```python
from build123d import *

# Parameters (mm, degrees)
SKETCH1_R           = 4.625
SKETCH1_R_2         = 1.625
BOSS_EXTRUDE1_DEPTH = 10
SKETCH1_3_R         = 19.75
SKETCH1_3_R_2       = 18.75
SKETCH1_3_R_3       = 17.65
SKETCH1_3_R_4       = 4.625
SKETCH1_3_R_5       = 15.65
SKETCH1_3_R_6       = 1.625
BOSS_EXTRUDE2_DEPTH = 5
SKETCH1_4_R         = 19.75
SKETCH1_4_R_2       = 18.75
SKETCH1_4_R_3       = 17.65
SKETCH1_4_R_4       = 15.65
BOSS_EXTRUDE3_DEPTH = 20
BOSS_EXTRUDE4_DEPTH = 20
SKETCH3_R           = 2
CUT_EXTRUDE1_DEPTH  = 35.352947472


with BuildPart() as part:
    # Sketch1 → Boss-Extrude1 (new body)
    with BuildSketch(Plane.XY):
        Circle(SKETCH1_R)
        Circle(SKETCH1_R_2, mode=Mode.SUBTRACT)
    extrude(amount=-BOSS_EXTRUDE1_DEPTH)



with BuildPart() as body_2:
    # Sketch1<3> → Boss-Extrude2 (new body)
    with BuildSketch(Plane.XY):
        Circle(SKETCH1_3_R)
        Circle(SKETCH1_3_R_2, mode=Mode.SUBTRACT)
        Circle(SKETCH1_3_R_2)
        Circle(SKETCH1_3_R_3, mode=Mode.SUBTRACT)
        Circle(SKETCH1_3_R_3)
        Circle(SKETCH1_3_R_4, mode=Mode.SUBTRACT)
        Circle(SKETCH1_3_R_5)
        Circle(SKETCH1_3_R_4, mode=Mode.SUBTRACT)
        Circle(SKETCH1_3_R_4)
        Circle(SKETCH1_3_R_6, mode=Mode.SUBTRACT)
    extrude(amount=BOSS_EXTRUDE2_DEPTH)


with BuildPart() as part_1:
    add(part.part)

    add(body_2.part)  # Boss-Extrude3 merges body 2
    # Sketch1<4> → Boss-Extrude3 (add)
    with BuildSketch(Plane.XY):
        Circle(SKETCH1_4_R)
        Circle(SKETCH1_4_R_2, mode=Mode.SUBTRACT)
        Circle(SKETCH1_4_R_3)
        Circle(SKETCH1_4_R_4, mode=Mode.SUBTRACT)
    extrude(amount=BOSS_EXTRUDE3_DEPTH)

    # Sketch2 → Boss-Extrude4 (add)
    with BuildSketch(Plane.XY):
        with BuildLine():
            Line((-4.757511558, 17.878182978), (-4.834765807, 18.115947107))
            ThreePointArc((-4.834765807, 18.115947107), (-5.794068645, 17.832309681), (-6.736878839, 17.497913119))
            Line((-6.736878839, 17.497913119), (-6.659624591, 17.260148989))
            Line((-6.659624591, 17.260148989), (-4.757511558, 17.878182978))
        make_face()
        with BuildLine():
            Line((-10.049324738, 15.533010498), (-10.196271051, 15.735264747))
            ThreePointArc((-10.196271051, 15.735264747), (-11.02097348, 15.169068645), (-11.814305039, 14.559694243))
            Line((-11.814305039, 14.559694243), (-11.667358726, 14.357439994))
            Line((-11.667358726, 14.357439994), (-10.049324738, 15.533010498))
        make_face()
        with BuildLine():
            Line((1, 18.473314343), (1, 18.723314343))
            ThreePointArc((1, 18.723314343), (0, 18.75), (-1, 18.723314343))
            Line((-1, 18.723314343), (-1, 18.473314343))
            Line((-1, 18.473314343), (1, 18.473314343))
        make_face()
        with BuildLine():
            Line((4.834765807, 18.115947107), (4.757511558, 17.878182978))
            Line((4.757511558, 17.878182978), (6.659624591, 17.260148989))
            Line((6.659624591, 17.260148989), (6.736878839, 17.497913119))
            ThreePointArc((6.736878839, 17.497913119), (5.794068645, 17.832309681), (4.834765807, 18.115947107))
        make_face()
        with BuildLine():
            ThreePointArc((11.814305039, 14.559694243), (11.02097348, 15.169068645), (10.196271051, 15.735264747))
            Line((10.196271051, 15.735264747), (10.049324738, 15.533010498))
            Line((10.049324738, 15.533010498), (11.667358726, 14.357439994))
            Line((11.667358726, 14.357439994), (11.814305039, 14.559694243))
        make_face()
        with BuildLine():
            ThreePointArc((15.735264747, 10.196271051), (15.169068645, 11.02097348), (14.559694243, 11.814305039))
            Line((14.559694243, 11.814305039), (14.357439994, 11.667358726))
            Line((14.357439994, 11.667358726), (15.533010498, 10.049324738))
            Line((15.533010498, 10.049324738), (15.735264747, 10.196271051))
        make_face()
        with BuildLine():
            ThreePointArc((18.115947107, 4.834765807), (17.832309681, 5.794068645), (17.497913119, 6.736878839))
            Line((17.497913119, 6.736878839), (17.260148989, 6.659624591))
            Line((17.260148989, 6.659624591), (17.878182978, 4.757511558))
            Line((17.878182978, 4.757511558), (18.115947107, 4.834765807))
        make_face()
        with BuildLine():
            ThreePointArc((18.75, 0), (18.743327399, 0.500177999), (18.723314343, 1))
            Line((18.723314343, 1), (18.473314343, 1))
            Line((18.473314343, 1), (18.473314343, -1))
            Line((18.473314343, -1), (18.723314343, -1))
            ThreePointArc((18.723314343, -1), (18.743327399, -0.500177999), (18.75, 0))
        make_face()
        with BuildLine():
            ThreePointArc((17.497913119, -6.736878839), (17.832309681, -5.794068645), (18.115947107, -4.834765807))
            Line((18.115947107, -4.834765807), (17.878182978, -4.757511558))
            Line((17.878182978, -4.757511558), (17.260148989, -6.659624591))
            Line((17.260148989, -6.659624591), (17.497913119, -6.736878839))
        make_face()
        with BuildLine():
            ThreePointArc((14.559694243, -11.814305039), (15.169068645, -11.02097348), (15.735264747, -10.196271051))
            Line((15.735264747, -10.196271051), (15.533010498, -10.049324738))
            Line((15.533010498, -10.049324738), (14.357439994, -11.667358726))
            Line((14.357439994, -11.667358726), (14.559694243, -11.814305039))
        make_face()
        with BuildLine():
            ThreePointArc((10.196271051, -15.735264747), (11.02097348, -15.169068645), (11.814305039, -14.559694243))
            Line((11.814305039, -14.559694243), (11.667358726, -14.357439994))
            Line((11.667358726, -14.357439994), (10.049324738, -15.533010498))
            Line((10.049324738, -15.533010498), (10.196271051, -15.735264747))
        make_face()
        with BuildLine():
            ThreePointArc((4.834765807, -18.115947107), (5.794068645, -17.832309681), (6.736878839, -17.497913119))
            Line((6.736878839, -17.497913119), (6.659624591, -17.260148989))
            Line((6.659624591, -17.260148989), (4.757511558, -17.878182978))
            Line((4.757511558, -17.878182978), (4.834765807, -18.115947107))
        make_face()
        with BuildLine():
            ThreePointArc((-1, -18.723314343), (0, -18.75), (1, -18.723314343))
            Line((1, -18.723314343), (1, -18.473314343))
            Line((1, -18.473314343), (-1, -18.473314343))
            Line((-1, -18.473314343), (-1, -18.723314343))
        make_face()
        with BuildLine():
            Line((-6.659624591, -17.260148989), (-6.736878839, -17.497913119))
            ThreePointArc((-6.736878839, -17.497913119), (-5.794068645, -17.832309681), (-4.834765807, -18.115947107))
            Line((-4.834765807, -18.115947107), (-4.757511558, -17.878182978))
            Line((-4.757511558, -17.878182978), (-6.659624591, -17.260148989))
        make_face()
        with BuildLine():
            Line((-11.667358726, -14.357439994), (-11.814305039, -14.559694243))
            ThreePointArc((-11.814305039, -14.559694243), (-11.02097348, -15.169068645), (-10.196271051, -15.735264747))
            Line((-10.196271051, -15.735264747), (-10.049324738, -15.533010498))
            Line((-10.049324738, -15.533010498), (-11.667358726, -14.357439994))
        make_face()
        with BuildLine():
            Line((-15.533010498, -10.049324738), (-15.735264747, -10.196271051))
            ThreePointArc((-15.735264747, -10.196271051), (-15.169068645, -11.02097348), (-14.559694243, -11.814305039))
            Line((-14.559694243, -11.814305039), (-14.357439994, -11.667358726))
            Line((-14.357439994, -11.667358726), (-15.533010498, -10.049324738))
        make_face()
        with BuildLine():
            Line((-17.878182978, -4.757511558), (-18.115947107, -4.834765807))
            ThreePointArc((-18.115947107, -4.834765807), (-17.832309681, -5.794068645), (-17.497913119, -6.736878839))
            Line((-17.497913119, -6.736878839), (-17.260148989, -6.659624591))
            Line((-17.260148989, -6.659624591), (-17.878182978, -4.757511558))
        make_face()
        with BuildLine():
            Line((-18.473314343, 1), (-18.723314343, 1))
            ThreePointArc((-18.723314343, 1), (-18.75, 0), (-18.723314343, -1))
            Line((-18.723314343, -1), (-18.473314343, -1))
            Line((-18.473314343, -1), (-18.473314343, 1))
        make_face()
        with BuildLine():
            Line((-14.357439994, 11.667358726), (-14.559694243, 11.814305039))
            ThreePointArc((-14.559694243, 11.814305039), (-15.169068645, 11.02097348), (-15.735264747, 10.196271051))
            Line((-15.735264747, 10.196271051), (-15.533010498, 10.049324738))
            Line((-15.533010498, 10.049324738), (-14.357439994, 11.667358726))
        make_face()
        with BuildLine():
            Line((-17.260148989, 6.659624591), (-17.497913119, 6.736878839))
            ThreePointArc((-17.497913119, 6.736878839), (-17.832309681, 5.794068645), (-18.115947107, 4.834765807))
            Line((-18.115947107, 4.834765807), (-17.878182978, 4.757511558))
            Line((-17.878182978, 4.757511558), (-17.260148989, 6.659624591))
        make_face()
    extrude(amount=BOSS_EXTRUDE4_DEPTH)

    # Sketch3 → Cut-Extrude1 (cut, through all)
    with BuildSketch(Plane(origin=(0, 0, 0), x_dir=(1, 0, 0), z_dir=(0, 1, 0))):
        with Locations(Location((0, 5, 0), (0, 0, 270))):
            Circle(SKETCH3_R)
    extrude(amount=-CUT_EXTRUDE1_DEPTH, mode=Mode.SUBTRACT)


solid = part_1.part
```
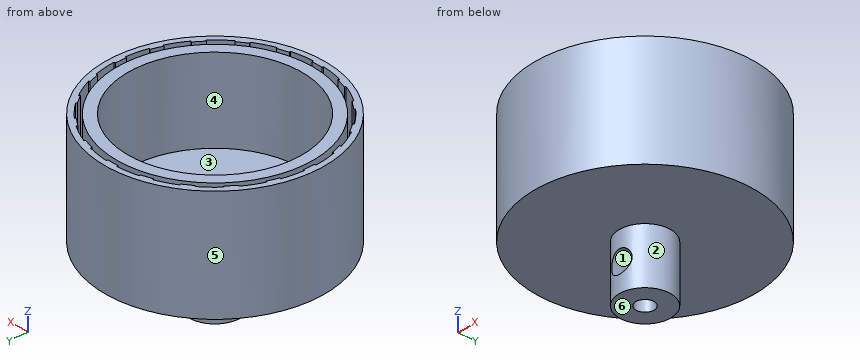
The listing builds one solid part. Answer for the finished solid, in the listing's coordinates (mm). Face numbers are marked on the shaded views. A direction names the side the tool comes from. Give positions to 0.01 mm unless a question says otherwise; leave off trailing zeros. Order: outer loops, then holes, each group sorted by start corner. A loop starts at its lowest first (then second) coordinate and runs counter-clockwise, first axis right, second up. Notation, with made-up numbers: (-37, 69.25) - (-28, 69.25) arc R22 ccw to (-28, 88.25) - close; hole circle Ø4 at (60, 41). An arc over 180 degrees is marked (long way). Answer in a Markdown table with one row per item. Add a question column.
Q1. The part is cut by section A-A (x = 0). Determine the outline of the cut face in (y, z) (3 decimals).
Q2. Given P1, Ø2, axis at x = -0.5, z = 14, coming from the +Y side; P2, Ø5, axis at y = 9, z = -3.5, coming from the -X side; P3, Ø8, axis at x = -11.5, z = -1, coming from the -Y side; P4, Ø6, axis at y = 13.5, z = 13, coming from the -X side, each flat-ended and moving along its own axis, determine where each tip first touches the part or whether it passes through.
Q3. The part is cut by section D-D (y = -6). Determine the outline of the cut face in (x, z), then the cut area to 3 significant figures.
Q4. The part is cut by section B-B (z = 6.5). Give the number of separate pieces and of enclosed holes in the cut face, then the cut area to 3 significant figures.
Q5. For a pull along Y with two mould halves and no side action, classify the marked faces 3, 4, 5 and 6 as released by +Y, released by -Y, zero draft, split by the parting line, or undercut.
Q6. Find the intervals of material crossed by line 1 along Y through (x, z) = (13, 18); line 2 along Y through (x, z) = (-8, 6.5); line 3 along X through (y, z) = (-4, 8.5), in increasing order. Write a range as [from, to].
Q7. The part is cut by section C-C (x = -13). Determine the outline of the cut face in (y, z).
Q8. Which of the six approach directions +Z, -Z, +X, -X, +Y, -Y give full straight-line access (tool end or side, diameter ignored) to the marked faces 1 and 2?
Determined:
| question | item | result |
|---|---|---|
| 1 | outline | (-19.75, 0) - (-4.625, 0) - (-4.625, -3) - (-1.625, -3) - (-1.625, 5) - (-15.65, 5) - (-15.65, 20) - (-17.65, 20) - (-17.65, 5) - (-18.473, 5) - (-18.473, 20) - (-19.75, 20) - close; (-4.625, -10) - (-1.625, -10) - (-1.625, -7) - (-4.625, -7) - close; (1.625, -10) - (4.625, -10) - (4.625, 0) - (19.75, 0) - (19.75, 20) - (18.473, 20) - (18.473, 5) - (17.65, 5) - (17.65, 20) - (15.65, 20) - (15.65, 5) - (1.625, 5) - close |
| 2 | P1 | stops at y = 19.75 |
| 2 | P2 | passes through |
| 2 | P3 | stops at y = -18.22 |
| 2 | P4 | stops at x = -16.73 |
| 3 | outline | (-18.82, 0) - (18.82, 0) - (18.82, 20) - (17.47, 20) - (17.47, 5) - (16.6, 5) - (16.6, 20) - (14.45, 20) - (14.45, 5) - (-14.45, 5) - (-14.45, 20) - (-16.6, 20) - (-16.6, 5) - (-17.47, 5) - (-17.47, 20) - (-18.82, 20) - close |
| 3 | area | 293 mm² |
| 4 | separate pieces | 2 |
| 4 | enclosed holes | 2 |
| 4 | area | 341 mm² |
| 5 | face 3 | undercut |
| 5 | face 4 | undercut |
| 5 | face 5 | split by the parting line |
| 5 | face 6 | zero draft |
| 6 | line 1 | y = [-14.87, -13.51], [-11.94, -8.71], [8.71, 11.94], [13.51, 14.87] |
| 6 | line 2 | y = [-18.06, -16.96], [-15.73, -13.45], [13.45, 15.73], [16.96, 18.06] |
| 6 | line 3 | x = [-19.34, -18.32], [-17.19, -15.13], [15.13, 17.19], [18.32, 19.34] |
| 7 | outline | (-14.87, 0) - (14.87, 0) - (14.87, 20) - (13.51, 20) - (13.51, 5) - (11.94, 5) - (11.94, 20) - (8.71, 20) - (8.71, 5) - (-8.71, 5) - (-8.71, 20) - (-11.94, 20) - (-11.94, 5) - (-13.51, 5) - (-13.51, 20) - (-14.87, 20) - close |
| 8 | face 1 | -Y |
| 8 | face 2 | -Z |
